Could you check a few things on this model? Use its own coordinates, in mm. Face numbers are marked on the shaded views. A direction names the side the tool comes from. Give positions to 0.01 mm unless a question says otherwise; leave off trailing zeros. Write each loop counter-clockwise with the first axis right and the second up, starting at its lowest first coordinate (ties: lowest second). Pieces come first, ordered by that corner, then holes. Notation, with made-up numbers: M 60,74 L 78,74 A22 cw 78,109 Z; hole C 65.25,11.25 d5. An arc over 180 degrees is marked long. One line per item, written item: value.
Autodesk Inventor part; units mm, degrees
ref_plane "YZ Plane" through (0, 0, 0) normal (1, 0, 0) x (0, 1, 0)
ref_plane "XZ Plane" through (0, 0, 0) normal (0, 1, 0) x (-1, 0, 0)
ref_plane "XY Plane" through (0, 0, 0) normal (0, 0, 1) x (1, 0, 0)
sketch "Sketch1" plane through (0, 0, 0) normal (1, 0, 0) x (0, 1, 0)
  line L0 (0, 0) -> (0, 32)
  arc A0 (0, 32) -> (0, 70) centre (0, 51) ccw
  line L1 (0, 70) -> (0, 107)
  line L2 (0, 0) -> (41, 0)
  line L3 (11, 107) -> (11, 78.9106)
  arc A1 (11, 23.0894) -> (11, 78.9106) centre (0, 51) ccw
  line L4 (11, 23.0894) -> (11, 11)
  line L5 (11, 11) -> (41, 11)
  line L6 (11, 107) -> (0, 107)
  line L7 (41, 11) -> (41, 0)
  dimension "d0" = 32
  dimension "d1" = 70
  dimension "d2" = 37
  dimension "d3" = 41
  dimension "d4" = 11
extrude "Extrusion1" add sketch "Sketch1" along normal blind 48
fillet "Fillet1" radius 13 1 edges at (48, 5.5, 107)
fillet "Fillet2" radius 13 1 edges at (0, 5.5, 107)
sketch "Sketch2" plane through (0, 11, 78.9106) normal (0, 1, 0) x (1, 0, 0)
  arc A0 (0, -15.0894) -> (13, -28.0894) centre (13, -15.0894) ccw
  circle A1 centre (13, -15.0894) radius 5
  arc A2 (35, -28.0894) -> (48, -15.0894) centre (35, -15.0894) ccw
  circle A3 centre (35, -15.0894) radius 5
  point P0 (0, 78.9106)
  dimension "d9" = 10
  dimension "d10" = 10
extrude "Extrusion2" cut sketch "Sketch2" against normal blind 11
fillet "Fillet3" radius 6 1 edges at (48, 41, 5.5)
fillet "Fillet4" radius 6 1 edges at (0, 41, 5.5)
sketch "Sketch3" plane through (48, 0, 0) normal (0, 0, -1) x (-1, 0, 0)
  line L0 (57.6, 0) -> (-9.6, 0) construction
  line L1 (48, -8.2) -> (48, 49.2)
  arc A0 (17.1801, 25) -> (30.1801, 25) centre (23.6801, 25) ccw
  line L2 (17.1801, 25) -> (17.1801, 41)
  line L3 (42, 41) -> (6, 41)
  line L4 (30.1801, 25) -> (30.1801, 41)
  point P0 (48, 0)
  dimension "d15" = 25
  dimension "d16" = 13
extrude "Extrusion3" cut sketch "Sketch3" against normal blind 11
sketch "Sketch4" plane through (0, 0, 0) normal (0, -1, 0) x (1, 0, 0)
  line L0 (0, 32) -> (48, 32)
  line L1 (0, 32) -> (0, 70)
  circle A0 centre (24, 51) radius 2.5
  point P0 (0, 0)
  point P1 (24, 32)
  point P2 (0, 51)
  dimension "d19" = 24
  dimension "d20" = 5
extrude "Extrusion4" cut sketch "Sketch4" against normal blind 41
properties part number "T05"
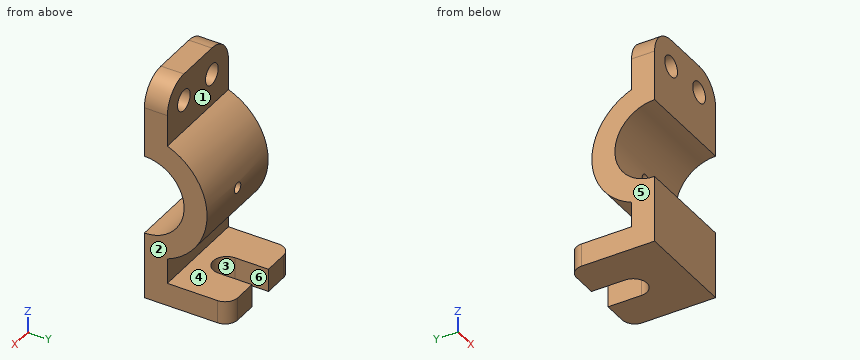
1) If we section it at A-A, the plane z = 51: Write out the boundary of the cut face in (x, y), then the cut area to 3 significant figures.
Outcome:
outline: M 0,19 L 21.5,19 L 21.5,30 L 0,30 Z; M 26.5,19 L 48,19 L 48,30 L 26.5,30 Z
area: 473 mm^2
2) If we section it at B-B, the plane y = 20: Write out the boundary of the cut face in (x, z).
Outcome:
outline: M 0,0 L 20.17,0 L 20.17,11 L 0,11 Z; M 0,28.64 L 48,28.64 L 48,73.36 L 0,73.36 Z; M 28.47,0 L 48,0 L 48,11 L 28.47,11 Z; hole C 24,51 d5
3) If we section it at D-D, the plane x = 38: Write out the boundary of the cut face in (y, z).
Outcome:
outline: M 0,0 L 41,0 L 41,11 L 11,11 L 11,23.09 A30 ccw 11,78.91 L 11,90 L 0,90 L 0,70 A19 cw 0,32 Z; M 0,98 L 11,98 L 11,106.65 L 0,106.65 Z
4) Please list where these lines run through material, in increasing order: L1, parallel to X at y = 7.75, z = 94; L2, parallel to X at y = 25, z = 51; L3, parallel to Z at x = 3, y = 31. Write a range as from..to.
Outcome:
L1: x = 0..8, 18..30, 40..48
L2: x = 0..21.5, 26.5..48
L3: z = 0..11
5) On a 3-axis mill with a long thin cutter (end or side, diameter ignored), from which of +Z, -Z, +X, -X, +Y, -Y can I reach the whole of each face in a straight line? I mean the marked faces 1, 2 and 3. Say none if no direction works.
Outcome:
face 1: +Z, +X, -X, +Y
face 2: +Z, -Z, +X, +Y, -Y
face 3: -Z, +Y
6) We'd pull the mould along X, two halves only. Please class the marked faces 4, 5 and 6: pulls with the +X half, pulls with the -X half, needs draft (parallel to the pull), parting line crosses it, or undercut.
Outcome:
face 4: needs draft
face 5: pulls with the -X half
face 6: undercut
7) If we section it at C-C, the plane y = 7: Write out the boundary of the cut face in (x, z).
Outcome:
outline: M 0,0 L 48,0 L 48,33.34 L 0,33.34 Z; M 0,68.66 L 48,68.66 L 48,94 A13 ccw 35,107 L 13,107 A13 ccw 0,94 Z; hole C 13,94 d10; hole C 35,94 d10
8) I'm going to push flat-ended pins straight in: pin 1 (1.5 mm diameter, centred on x = 30.5, z = 27.5, fed in from +Y); pin 2 (9 mm diameter, centred on x = 18.5, y = 23, fed in from +Z); pin 3 (14 mm diameter, centred on x = 21, z = 95, fed in from +Y). Where does each tip first touch, or does it pass through?
Outcome:
pin 1: stops at y = 19.56
pin 2: stops at z = 74.62
pin 3: stops at y = 11
